from build123d import *

# Parameters (mm, degrees)
SKETCH1_W                      = 30
SKETCH1_H                      = 60
BOSS_EXTRUDE1_DEPTH            = 6.35
CBORE_FOR_M4_SHCS1_D           = 4.8
CBORE_FOR_M4_SHCS1_DEPTH       = 6.35
CBORE_FOR_M4_SHCS1_CBORE_D     = 8
CBORE_FOR_M4_SHCS1_CBORE_DEPTH = 4
SKETCH4_W                      = 6.35
SKETCH4_H                      = 15
CUT_EXTRUDE1_DEPTH             = 7.35
SKETCH5_R                      = 1
CUT_EXTRUDE2_DEPTH             = 7.35
FILLET1_R                      = 1
FILLET2_R                      = 2


with BuildPart() as part:
    # Sketch1 → Boss-Extrude1 (new body)
    with BuildSketch(Plane(origin=(0, 0, 0), x_dir=(1, 0, 0), z_dir=(0, 1, 0))):
        Rectangle(SKETCH1_W, SKETCH1_H)
    extrude(amount=BOSS_EXTRUDE1_DEPTH)

    # CBORE for M4 SHCS1
    with Locations(Plane(origin=(0, 6.35, 0), x_dir=(1, 0, 0), z_dir=(0, 1, 0))):
        with Locations((-5, 20), (-5, -20)):
            CounterBoreHole(CBORE_FOR_M4_SHCS1_D / 2, CBORE_FOR_M4_SHCS1_CBORE_D / 2, CBORE_FOR_M4_SHCS1_CBORE_DEPTH, depth=CBORE_FOR_M4_SHCS1_DEPTH)

    # Sketch4 → Cut-Extrude1 (cut, through all)
    with BuildSketch(Plane(origin=(0, 6.35, 0), x_dir=(1, 0, 0), z_dir=(0, 1, 0))):
        with Locations((6.825, 17.5)):
            Rectangle(SKETCH4_W, SKETCH4_H)
    cut_extrude1 = extrude(amount=-CUT_EXTRUDE1_DEPTH, mode=Mode.SUBTRACT)

    # Sketch5 → Cut-Extrude2 (cut, through all)
    with BuildSketch(Plane(origin=(0, 6.35, 0), x_dir=(1, 0, 0), z_dir=(0, 1, 0))):
        with Locations((3.65, 25)):
            Circle(SKETCH5_R)
        with Locations((10, 25)):
            Circle(SKETCH5_R)
        with Locations((10, 10)):
            Circle(SKETCH5_R)
        with Locations((3.65, 10)):
            Circle(SKETCH5_R)
    cut_extrude2 = extrude(amount=-CUT_EXTRUDE2_DEPTH, mode=Mode.SUBTRACT)

    # Mirror1: Cut-Extrude1, Cut-Extrude2 across plane
    add(cut_extrude1.mirror(Plane.XY), mode=Mode.SUBTRACT)
    add(cut_extrude2.mirror(Plane.XY), mode=Mode.SUBTRACT)

    # Fillet1
    fillet1_edges = [part.edges().sort_by_distance(p)[0] for p in [
        (9, 3.175, 25),
        (10, 3.175, 11),
        (4.65, 3.175, 10),
        (3.65, 3.175, 11),
        (9, 3.175, 10),
        (10, 3.175, 24),
        (3.65, 3.175, 24),
        (9, 3.175, -10),
        (4.65, 3.175, -10),
        (10, 3.175, -24),
        (4.65, 3.175, -25),
        (3.65, 3.175, -11),
        (10, 3.175, -11),
        (9, 3.175, -25),
        (3.65, 3.175, -24),
        (4.65, 3.175, 25),
    ]]
    fillet(fillet1_edges, radius=FILLET1_R)

    # Fillet2
    fillet2_edges = [part.edges().sort_by_distance(p)[0] for p in [
        (-15, 3.175, -30),
        (15, 3.175, -30),
        (15, 3.175, 30),
        (-15, 3.175, 30),
    ]]
    fillet(fillet2_edges, radius=FILLET2_R)


solid = part.part
Verification items for the finished model (mm, model axes). A direction names the side the tool comes from. Coordinates: 2 decimals unless noted, no trailing zeros. Order: outer loops, then holes, each group sorted by start corner. A loop starts at its lowest first (then second) coordinate and runs counter-clockwise, first axis right, second up. Notation, with made-up numbers: (-38.75, 31) -> (4.25, 31) arc R28 cw to (4.25, 60) -> close; hole circle Ø3 at (29.25, 17). An arc over 180 degrees is marked (long way). Use CSV: the item, a comma, the result in double quotes. Start each with the question number.
Q1. Thickness scan on line 1 along Z through (x, y) = (-5, 4.5); line 2 along Z through (x, y) = (5, 5); line 3 along X through (y, z) = (4.75, 9.5). Record the ranges inside material, lowest first.
Q2. Section check A-A, the plane x = -5. Record the cut outline in (y, z), and give its area (3 significant figures).
Q3. Tool access check on faces 1 (the flat face through (-3, 2.35, -18)), 2 (the flat face through (10, 3, 17)), 3 (the cylindrical face through (-14.43, 3.22, -29.4)). Record the directions out of +Z, -Z, +X, -X, +Y, -Y that give a thin tool (end or side, any length) a straight path to the whole face; none if there is none.
Q4. Section check B-B, the plane z = 20. Record the cut outline in (x, y).
Q5. Depth check by flat-ended pin: P1, Ø2.5, axis at x = -6.5, z = -20.5, coming from the +Y side; P2, Ø9, axis at x = -5.5, z = 20.5, coming from the +Y side. Enter the tip coordinate at first touch or a pass-through.
Q6. Section check C-C, the plane y = 3.75. Give the number of separate pieces and of enclosed holes in the cut face, and give its area (3 significant figures).
Q7. Draft check along Z on faces 4 (the flat face through (0, 6.35, 0)), 5 (the flat face through (0, 3, -30)), 6 (the flat face through (7, 3, 25)). Enter one of: +Z half, -Z half, draft (parallel to the pull), parting line (faces both ways), or undercut.
Returned:
1,line 1,"z = -30 to -24, -16 to 16, 24 to 30"
1,line 2,"z = -30 to -25.08, -9.92 to 9.92, 25.08 to 30"
1,line 3,"x = -15 to 2.78, 4.52 to 9.13, 10.87 to 15"
2,outline,"(0, -30) -> (6.35, -30) -> (6.35, -24) -> (2.35, -24) -> (2.35, -22.4) -> (0, -22.4) -> close; (0, -17.6) -> (2.35, -17.6) -> (2.35, -16) -> (6.35, -16) -> (6.35, 16) -> (2.35, 16) -> (2.35, 17.6) -> (0, 17.6) -> close; (0, 22.4) -> (2.35, 22.4) -> (2.35, 24) -> (6.35, 24) -> (6.35, 30) -> (0, 30) -> close"
2,area,"294 mm^2"
3,face 1,"+Y"
3,face 2,"+Y, -Y"
3,face 3,"-Z, -X, +Y, -Y"
4,outline,"(-15, 0) -> (-7.4, 0) -> (-7.4, 2.35) -> (-9, 2.35) -> (-9, 6.35) -> (-15, 6.35) -> close; (-2.6, 0) -> (3.65, 0) -> (3.65, 6.35) -> (-1, 6.35) -> (-1, 2.35) -> (-2.6, 2.35) -> close; (10, 0) -> (15, 0) -> (15, 6.35) -> (10, 6.35) -> close"
5,P1,"stops at y = 2.35"
5,P2,"stops at y = 6.35"
6,separate pieces,"1"
6,enclosed holes,"4"
6,area,"1,490 mm^2"
7,face 4,"draft"
7,face 5,"-Z half"
7,face 6,"undercut"
